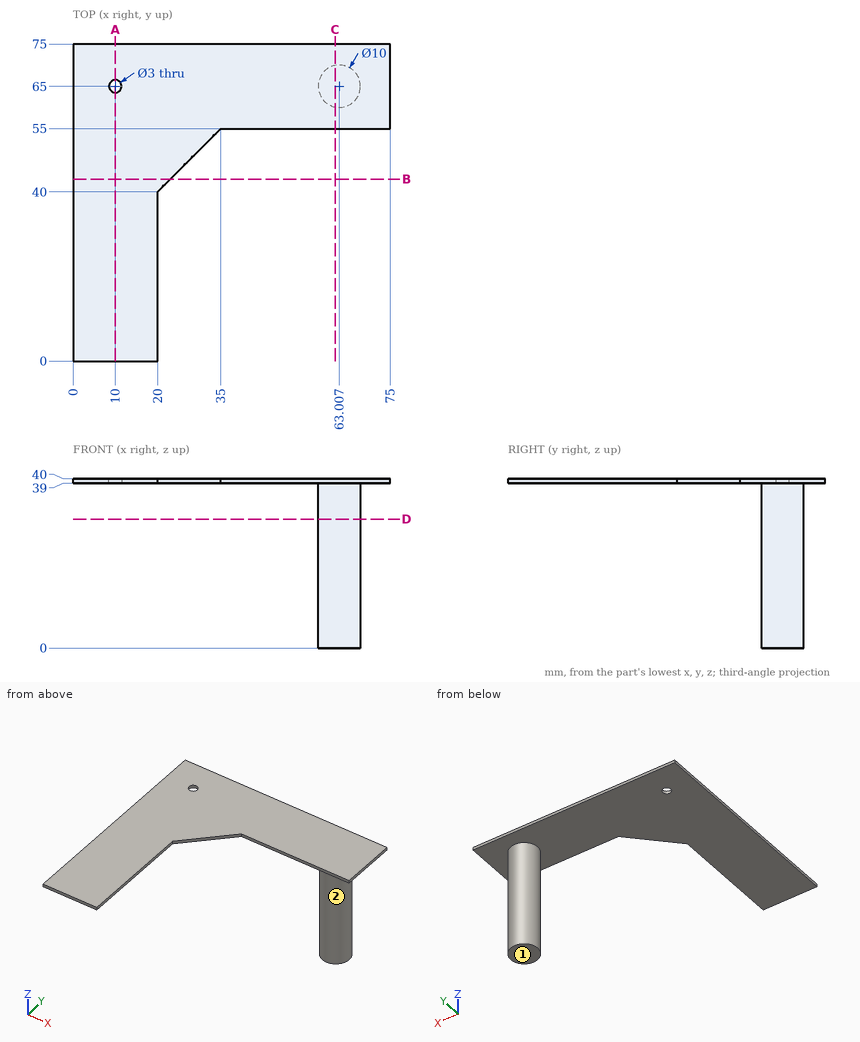
Print and shaded views of the part. All mm, measured from the part's lowest x, y and z. A direction names the side the tool comes from. Coordinates: 2 decimals unless noted, no trailing zeros. Write each loop counter-clockwise with the first axis right and the second up, starting at its lowest first coordinate (ties: lowest second). Pieces come first, ordered by that corner, then holes. Notation, with made-up numbers: (32, 11) - (54, 11) arc R20 cw to (54, 16) - close; hole circle Ø2 at (10, 17). An arc over 180 degrees is marked (long way). One line per question, with ' | ' between items. Start each with the question number.
Q1. 3-axis set-ups, long thin cutter, end or side, ignore diameter. For the marked faces 1 and 2: which of +Z, -Z, +X, -X, +Y, -Y reach the whole face in a straight line?
Q2. Drill centre line: line 1 (Z direction, x = 12, y = 13). Where is it in solid material? Low to high. Write a range as [from, to].
Q3. Cut at C-C, the plane x = 62. List the corners of the cut face in (y, z).
Q4. Pin check, flat tips, straight feed: pin 1 (2.5 mm diameter, centred on x = 10, y = 65, fed in from +Z); pin 2 (4 mm diameter, centred on x = 66, z = 29.5, fed in from -Y); pin 3 (10 mm diameter, centred on x = 57.5, z = 6.5, fed in from -Y); pin 4 (1.5 mm diameter, centred on x = 24.5, y = 47, fed in from -Z). Stop position of each tip, or through.
Q5. Cut at A-A, the plane x = 10. List the corners of the cut face in (y, z).
Q6. Cut at D-D, the plane z = 30.5. List the corners of the cut face in (x, y).
Q7. Cut at B-B, the plane y = 43. List the corners of the cut face in (x, z), then the cut area to 3 significant figures.
Answer below:
1) face 1: -Z, +X, -X, +Y, -Y | face 2: -Z
2) line 1: [39, 40]
3) outline: (55, 39) - (60.1, 39) - (60.1, 0) - (69.9, 0) - (69.9, 39) - (75, 39) - (75, 40) - (55, 40) - close
4) pin 1: through | pin 2: y = 60.1 | pin 3: y = 60.03 | pin 4: z = 39
5) outline: (0, 39) - (63.5, 39) - (63.5, 40) - (0, 40) - close; (66.5, 39) - (75, 39) - (75, 40) - (66.5, 40) - close
6) outline: circle Ø10 at (63.01, 65)
7) outline: (0, 39) - (23, 39) - (23, 40) - (0, 40) - close | area: 23.0 mm^2
